from build123d import *

# Parameters (mm, degrees)
F0_W     = 78.8246691227
F0_H     = 118.5333281755
F1_DEPTH = 25.4
F2_R     = 38.1
F3_R     = 15.1432948242
F4_DEPTH = 25.401
F5_W     = 78.8246691227
F5_H     = 20.3456624932
F6_DEPTH = 58.42
F7_W     = 19.0527010709
F7_H     = 20.3456624932
F8_DEPTH = 19.558


with BuildPart() as f1:
    # F0 (on Front) → F1 (new body)
    with BuildSketch(Plane.XZ):
        Rectangle(F0_W, F0_H)
    extrude(amount=F1_DEPTH)

    # F2
    f2_edges = [f1.edges().sort_by_distance(p)[0] for p in [
        (-39.412335, -12.7, 59.266664),
        (39.412335, -12.7, 59.266664),
    ]]
    fillet(f2_edges, radius=F2_R)

    # F3 (on Front) → F4 (cut, through all)
    with BuildSketch(Plane.XZ):
        with Locations((0, 30.226001516)):
            Circle(F3_R)
    extrude(amount=F4_DEPTH, mode=Mode.SUBTRACT)

    # F5 (on Front) → F6 (join)
    with BuildSketch(Plane.XZ):
        with Locations((0, -49.0938328412)):
            Rectangle(F5_W, F5_H)
    extrude(amount=-F6_DEPTH)

    # F7 (on face) → F8 (cut)
    with BuildSketch(Plane(origin=(0, 58.42, 0), x_dir=(-1, 0, 0), z_dir=(0, 1, 0))):
        with Locations((29.8859840259, -49.0938328412)):
            Rectangle(F7_W, F7_H)
    extrude(amount=-F8_DEPTH, mode=Mode.SUBTRACT)


solid = f1.part
Check sheet for the modelled part. Datum: model origin and axes. Units: mm. A direction names the side the tool comes from. Give positions to 0.01 mm unless a question says otherwise; leave off trailing zeros. Order: outer loops, then holes, each group sorted by start corner. A loop starts at its lowest first (then second) coordinate and runs counter-clockwise, first axis right, second up. Notation, with made-up numbers: (8.5, -40) - (59.5, -40) arc R20 cw to (59.5, -21) - close; hole circle Ø7 at (52, -6.5). An arc over 180 degrees is marked (long way). Answer as CSV lines item,"result".
1. Tool access check on faces 4 (the face through (-1, 0, 0)), 5 (the face through (39.412, -3, -29)), 6 (the face through (-30, 38.862, -49)). Record the directions out of +Z, -Z, +X, -X, +Y, -Y that give a thin tool (end or side, any length) a straight path to the whole face; none if there is none.
Result sheet:
face 4,"+Z, +X, -X, +Y"
face 5,"+Z, -Z, +X, +Y, -Y"
face 6,"+Z, -Z, -X, +Y"
2. Section check A-A (z = 37.5). Record the boundary of the cut face in (x, y).
Result sheet:
outline,"(-35.73, -25.4) - (-13.28, -25.4) - (-13.28, 0) - (-35.73, 0) - close; (13.28, -25.4) - (35.73, -25.4) - (35.73, 0) - (13.28, 0) - close"
3. Section check D-D (y = 8.5). Record the boundary of the cut face in (x, z).
Result sheet:
outline,"(-39.41, -59.27) - (39.41, -59.27) - (39.41, -38.92) - (-39.41, -38.92) - close"
4. Section check C-C (y = -8.5). Record the boundary of the cut face in (x, z).
Result sheet:
outline,"(-39.41, -59.27) - (39.41, -59.27) - (39.41, 21.17) arc R38.1 ccw to (1.31, 59.27) - (-1.31, 59.27) arc R38.1 ccw to (-39.41, 21.17) - close; hole circle Ø30.29 at (0, 30.23)"
5. Mould release check, pull along Z, two halves, no side actions. Record for faces 1 (the face through (-1, 16, -59.267)), 2 (the face through (-1.97, -12.52, 45.24)), 3 (the face through (28.55, -12.88, 47.81)): released by +Z, released by -Z, zero draft, split by the parting line, or undercut.
Result sheet:
face 1,"released by -Z"
face 2,"undercut"
face 3,"released by +Z"
6. Go/stop test with flat-tipped pins: P1, Ø21, axis at x = -33, z = -46, coming from the +Y side; P2, Ø5, axis at x = -28.5, z = 37.5, coming from the +Y side; P3, Ø10, axis at y = 46.5, z = -45, coming from the -X side. Record where each tip stops, or that it passes through.
Result sheet:
P1,"y = 38.86"
P2,"y = 0"
P3,"x = -20.36"
7. Section check B-B (x = -9). Record the boundary of the cut face in (y, z), then the cut area to 3 significant figures.
Result sheet:
outline,"(-25.4, -59.27) - (58.42, -59.27) - (58.42, -38.92) - (0, -38.92) - (0, 18.05) - (-25.4, 18.05) - close; (-25.4, 42.4) - (0, 42.4) - (0, 58.48) - (-25.4, 58.48) - close"
area,"3,560 mm²"
8. Scan lines: probe 1 along Z at (x, y) = (0, -9); probe 2 along X at (y, z) = (46, -51); probe 3 along Y at (x, z) = (-35, 34). Record each from-to range of solid material in increasing order. Write a range as from..to.
Result sheet:
probe 1,"-59.27..15.08, 45.37..59.27"
probe 2,"-20.36..39.41"
probe 3,"-25.4..0"
